Verification items for the finished model (mm, model axes). Round coordinates to 2 decimals unless told otherwise and drop trailing zeros. Order: outer loops, then holes, each group sorted by start corner. A loop starts at its lowest first (then second) coordinate and runs counter-clockwise, first axis right, second up. Notation, with made-up numbers: M 57.5,27 L 84.5,27 A16 cw 84.5,48 Z; hole C 80.5,-36.75 d2. An arc over 180 degrees is marked long. Use CSV: the item, a comma, the result in double quotes. Start each with the question number.
Q1. Sectioned sample at A-A (y = 16). Enter the section's corners in (x, z), and give its area (3 significant figures).
Q2. Sectioned sample at B-B (z = 804.5). Enter the section's corners in (x, y), and give its area (3 significant figures).
Q3. Sectioned sample at C-C (x = 12.5). Enter the section's corners in (y, z), and give its area (3 significant figures).
Q4. Scan lines: line 1 (X direction, y = 29, z = 193); line 2 (X direction, y = 28, z = 1004). Record each from-to range of solid material in increasing order.
Q5. Gauge pin test, flat end, axial feed: pin 1 Ø10 at (x, y) = (22.5, -25.5) entering from +Z. Record the tip position at first contact, or that the pin passes through.
Autodesk Inventor part; units mm, degrees
ref_plane "Start Plane" through (0, 0, 57.9828) normal (0, 0, 1) x (1, 0, 0)
ref_plane "End Plane" through (0, 0, 1356.2308) normal (0, 0, 1) x (1, 0, 0)
ref_plane "Work Plane4" through (-678.1154, 28, 678.1154) normal (-0.7071, 0, 0.7071) x (0.7071, 0, 0.7071)
ref_plane "Start Plane" through (0, 0, 57.9828) normal (0, 0, 1) x (1, 0, 0)
ref_plane "End Plane" through (0, 0, 1356.2308) normal (0, 0, 1) x (1, 0, 0)
sketch "Sketch" plane through (0, 0, 0) normal (0, 0, 1) x (1, 0, 0)
  line L0 (-40, -28) -> (-40, 28)
  line L1 (-28, 40) -> (28, 40)
  line L2 (40, 28) -> (40, -28)
  line L3 (28, -40) -> (-28, -40)
  arc A0 (-40, -28) -> (-28, -40) centre (-28, -28) ccw
  arc A1 (-28, 40) -> (-40, 28) centre (-28, 28) ccw
  arc A2 (40, 28) -> (28, 40) centre (28, 28) ccw
  arc A3 (28, -40) -> (40, -28) centre (28, -28) ccw
  arc A4 (-28, 32) -> (-32, 28) centre (-28, 28) ccw
  line L4 (-28, 32) -> (28, 32)
  arc A5 (32, 28) -> (28, 32) centre (28, 28) ccw
  line L5 (32, 28) -> (32, -28)
  arc A6 (28, -32) -> (32, -28) centre (28, -28) ccw
  line L6 (28, -32) -> (-28, -32)
  arc A7 (-32, -28) -> (-28, -32) centre (-28, -28) ccw
  line L7 (-32, -28) -> (-32, 28)
  line L8 (0, 59.4794) -> (0, -59.4794) construction
  line L9 (-59.4794, 0) -> (59.4794, 0) construction
  dimension "d7" = 12
  dimension "d10" = 80
  dimension "d11" = 80
  dimension "d12" = 8
  dimension "d15" = 40
  dimension "d16" = 40
extrude "Body" add sketch "Sketch" along normal up to surface (1298.2481 mm away) from surface at 57.9828
sketch "Sketch3" plane through (0, 0, 0) normal (0, 0, 1) x (1, 0, 0)
  line L0 (0, 0) -> (10, 0)
ref_plane "Work Plane3" through (0, 0, 0) normal (0, -1, 0) x (1, 0, 0)
ref_plane "Work Plane4" through (-678.1154, 28, 678.1154) normal (-0.7071, 0, 0.7071) x (0.7071, 0, 0.7071)
split "Split1" plane through (-678.1154, 28, 678.1154) removes the side toward (-0.7071, 0, 0.7071)
ref_plane "Work Plane5" through (678.1154, 28, 736.0982) normal (0.7071, 0, -0.7071) x (-0.7071, 0, -0.7071)
split "Split2" plane through (678.1154, 28, 736.0982) removes the side toward (0.7071, 0, -0.7071)
ref_plane "Work Plane6" through (-28.9914, 28, 1385.2222) normal (0.7071, 0, 0.7071) x (0.7071, 0, -0.7071)
split "Split3" plane through (-28.9914, 28, 1385.2222) removes the side toward (0.7071, 0, 0.7071)
ref_plane "Work Plane7" through (-678.1154, -28, 736.0982) normal (-0.7071, 0, -0.7071) x (-0.7071, 0, 0.7071)
split "Split4" plane through (-678.1154, -28, 736.0982) removes the side toward (-0.7071, 0, -0.7071)
sketch "Sketch4" plane through (0, 0, 0) normal (0, -1, 0) x (1, 0, 0)
  line L0 (-2, 57.9828) -> (12, 57.9828)
  line L1 (-2, 1356.2308) -> (12, 1356.2308)
  dimension "d18" = 1298.248
equation "\"d7\" = G_IR"
equation "\"d10\" = G_H"
equation "\"d11\" = G_W"
equation "\"d12\" = G_T"
equation "\"d15\" = 0.5 * d10"
equation "\"d16\" = 0.5 * d11"
equation "\"d3\" = G_L"
equation "\"G_W\" = 80"
equation "\"G_H\" = 80"
equation "\"G_T\" = 8"
equation "\"G_IR\" = 12"
equation "\"G_L\" = d18"
equation "\"G_OFFSET_START\" = -57.98276"
equation "\"G_OFFSET_END\" = -57.98276"
equation "\"d13\" = -G_OFFSET_START"
equation "\"d14\" = G_OFFSET_END + B_L"
equation "\"B_L\" = 1414.21356"
properties part number "ISO 12633-2 - 80x80x8 - 1298.25" material "Steel, Mild"
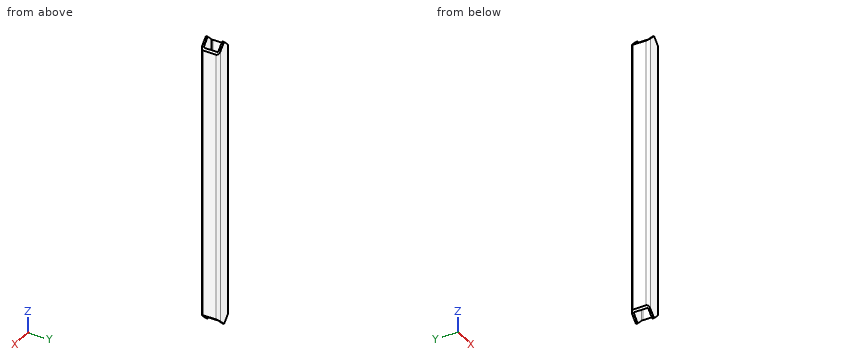
Verdict:
1,outline,"M -40,97.98 L -32,89.98 L -32,1324.23 L -40,1316.23 Z; M 32,89.98 L 40,97.98 L 40,1316.23 L 32,1324.23 Z"
1,area,"19,600 mm²"
2,outline,"M -40,-28 A12 ccw -28,-40 L 28,-40 A12 ccw 40,-28 L 40,28 A12 ccw 28,40 L -28,40 A12 ccw -40,28 Z; hole M -32,-28 A4 ccw -28,-32 L 28,-32 A4 ccw 32,-28 L 32,28 A4 ccw 28,32 L -28,32 A4 ccw -32,28 Z"
2,area,"2,190 mm²"
3,outline,"M -40,70.48 L -32,70.48 L -32,1343.73 L -40,1343.73 Z; M 32,70.48 L 40,70.48 L 40,1343.73 L 32,1343.73 Z"
3,area,"20,400 mm²"
4,line 1,"x = -39.96 to -31.87, 31.87 to 39.96"
4,line 2,"x = -40 to -32, 32 to 40"
5,pin 1,"passes through"
